Check sheet for the modelled part. Datum: model origin and axes. Units: mm. A direction names the side the tool comes from. Give positions to 0.01 mm unless a question says otherwise; leave off trailing zeros. Order: outer loops, then holes, each group sorted by start corner. A loop starts at its lowest first (then second) coordinate and runs counter-clockwise, first axis right, second up.
```python
from build123d import *

# Parameters (mm, degrees)
SZKIC1_W                     = 60
SZKIC1_H                     = 60
DODANIE_WYCI_GNI_CIE1_DEPTH  = 36.75
SFAZOWANIE1_SIZE             = 5
SFAZOWANIE2_SIZE             = 1
OTW_R_POD_RUB_M51_AT_2_COUNT = 2
OTW_R_POD_RUB_M51_AT_2_PITCH = 47.14
OTW_R_POD_RUB_M51_AT_3_COUNT = 2
OTW_R_POD_RUB_M51_AT_3_PITCH = 66.66602733
OTW_R_POD_RUB_M51_AT_4_COUNT = 2
OTW_R_POD_RUB_M51_AT_4_PITCH = 47.14


with BuildPart() as part:
    # Szkic1 → Dodanie-wyciągnięcie1 (new, symmetric)
    with BuildSketch(Plane(origin=(0, 0, 0), x_dir=(1, 0, 0), z_dir=(0, 1, 0))):
        Rectangle(SZKIC1_W, SZKIC1_H)
    extrude(amount=DODANIE_WYCI_GNI_CIE1_DEPTH, both=True)

    # Szkic2 → Wycięcie-obrót1 (revolve, cut)
    with BuildSketch(Plane.XY, mode=Mode.PRIVATE) as wyci_cie_obr_t1_sk:
        Polygon((29, 4.017949192), (30, 5.75), (36.080330081, 16.281440627), (59, 16.281440627), (59, -27.714101615), (30, -27.714101615), (29, -25.982050808), align=None)
    revolve(wyci_cie_obr_t1_sk.sketch.rotate(Axis((0, 0, 0), (0, 1, 0)), 90), axis=Axis((0, 0, 0), (0, 1, 0)), mode=Mode.SUBTRACT)

    # Sfazowanie1
    sfazowanie1_edges = [part.edges().sort_by_distance(p)[0] for p in [
        (30, -32.232050808, 30),
        (-30, -32.232050808, 30),
        (-30, -32.232050808, -30),
        (30, -32.232050808, -30),
        (30, 26.515720314, 30),
        (-30, 26.515720314, 30),
        (-30, 26.515720314, -30),
        (30, 26.515720314, -30),
    ]]
    chamfer(sfazowanie1_edges, length=SFAZOWANIE1_SIZE)

    # Szkic4 → Wycięcie-obrót3 (revolve, cut)
    with BuildSketch(Plane.XY, mode=Mode.PRIVATE) as wyci_cie_obr_t3_sk:
        Polygon((0, 36.75), (19.05, 36.75), (19.05, 31.75), (4, 31.75), (4, 16.75), (0, 16.75), align=None)
    revolve(wyci_cie_obr_t3_sk.sketch.rotate(Axis((0, 0, 0), (0, 1, 0)), 90), axis=Axis((0, 0, 0), (0, 1, 0)), mode=Mode.SUBTRACT)

    # Szkic5 → Obrót1 (revolve)
    with BuildSketch(Plane(origin=(0, 0, 0), x_dir=(0, 0, -1), z_dir=(1, 0, 0)), mode=Mode.PRIVATE) as obr_t1_sk:
        Polygon((0, -36.75), (20, -36.75), (20, -39.25), (9, -39.25), (9, -40.75), (7, -40.75), (7, -71.75), (0, -71.75), align=None)
    revolve(obr_t1_sk.sketch.rotate(Axis((0, 0, 0), (0, -1, 0)), 180), axis=Axis((0, 0, 0), (0, -1, 0)))

    # Sfazowanie2
    sfazowanie2_edges = [part.edges().sort_by_distance(p)[0] for p in [
        (0, -71.75, -7),
    ]]
    chamfer(sfazowanie2_edges, length=SFAZOWANIE2_SIZE)

    # Szkic7 → Otwór pod śrubę M51 (revolve, cut)
    with BuildSketch(Plane(origin=(23.57, -36.75, -23.57), x_dir=(0, 0, -1), z_dir=(1, 0, 0))):
        Polygon((0, 0), (0, 12.652366702), (2.75, 11), (2.75, 0), align=None)
    otw_r_pod_rub_m51 = revolve(axis=Axis((23.57, -43.1, -23.57), (0, 1, 0)), mode=Mode.SUBTRACT)

    # Otwór pod śrubę M51 at 2: Otwór pod śrubę M51 ×2
    with Locations(*[(-i * OTW_R_POD_RUB_M51_AT_2_PITCH, 0, 0) for i in range(1, OTW_R_POD_RUB_M51_AT_2_COUNT)]):
        add(otw_r_pod_rub_m51, mode=Mode.SUBTRACT)

    # Otwór pod śrubę M51 at 3: Otwór pod śrubę M51 ×2
    with Locations(*[Vector(-0.7071067811865477, 0, 0.7071067811865475) * (i * OTW_R_POD_RUB_M51_AT_3_PITCH) for i in range(1, OTW_R_POD_RUB_M51_AT_3_COUNT)]):
        add(otw_r_pod_rub_m51, mode=Mode.SUBTRACT)

    # Otwór pod śrubę M51 at 4: Otwór pod śrubę M51 ×2
    with Locations(*[(0, 0, i * OTW_R_POD_RUB_M51_AT_4_PITCH) for i in range(1, OTW_R_POD_RUB_M51_AT_4_COUNT)]):
        add(otw_r_pod_rub_m51, mode=Mode.SUBTRACT)

    # Lustro1: Otwór pod śrubę M51 across plane
    add(otw_r_pod_rub_m51.mirror(Plane.ZX), mode=Mode.SUBTRACT)

    # Lustro1 copy 1 sketch → Lustro1 copy 1 (revolve, cut)
    with BuildSketch(Plane(origin=(-23.57, 36.75, -23.57), x_dir=(0, 0, -1), z_dir=(1, 0, 0))):
        Polygon((0, 0), (0, -12.652366702), (2.75, -11), (2.75, 0), align=None)
    revolve(axis=Axis((-23.57, 43.1, -23.57), (0, 1, 0)), mode=Mode.SUBTRACT)

    # Lustro1 copy 2 sketch → Lustro1 copy 2 (revolve, cut)
    with BuildSketch(Plane(origin=(-23.57, 36.75, 23.57), x_dir=(0, 0, -1), z_dir=(1, 0, 0))):
        Polygon((0, 0), (0, -12.652366702), (2.75, -11), (2.75, 0), align=None)
    revolve(axis=Axis((-23.57, 43.1, 23.57), (0, 1, 0)), mode=Mode.SUBTRACT)

    # Lustro1 copy 3 sketch → Lustro1 copy 3 (revolve, cut)
    with BuildSketch(Plane(origin=(23.57, 36.75, 23.57), x_dir=(0, 0, -1), z_dir=(1, 0, 0))):
        Polygon((0, 0), (0, -12.652366702), (2.75, -11), (2.75, 0), align=None)
    revolve(axis=Axis((23.57, 43.1, 23.57), (0, 1, 0)), mode=Mode.SUBTRACT)


solid = part.part
```
(1) Material ranges on L1, parallel to X at y = 33, z = -23.57; L2, parallel to X at y = -30, z = 24, recorded low to high.
Response values:
L1: x = -30 to -26.32, -20.82 to 20.82, 26.32 to 30
L2: x = -30 to -26.29, -20.85 to 20.85, 26.29 to 30
(2) Cross-section at A-A on y = -8.5. Enter the section's corners in (x, z), then the cut area to 3 significant figures.
Response values:
outline: circle Ø58 at (0, 0)
area: 2,640 mm2
(3) Set-up check for faces 1 (the face through (20.843, -32.295, -23.212)), 2 (the face through (0, -71.75, 0)), 3 (the face through (-27, 16.281, -27)), 4 (the face through (-14, 36.75, -14)), 5 (the face through (-5, 31.75, 0)): record each of +Z, -Z, +X, -X, +Y, -Y from which the full face is reachable in a straight line by a thin tool's end or side.
Response values:
face 1: -Y
face 2: +Z, -Z, +X, -X, -Y
face 3: -Z, -X
face 4: +Z, -Z, +X, -X, +Y
face 5: +Y
(4) Gauge pin test, flat ends, axial feed: pin 1 Ø12 at (x, z) = (17.5, -12) entering from -Y; pin 2 Ø5 at (x, z) = (27.5, 26.5) entering from -Y; pin 3 Ø3.5 at (x, z) = (-23.57, -23.57) entering from +Y; pin 4 Ø20 at (x, z) = (10, -3) entering from -Y. Record the tip position at first contact, or that the pin passes through.
Response values:
pin 1: stops at y = -39.25
pin 2: stops at y = -36.75
pin 3: stops at y = 25.15
pin 4: stops at y = -71.75
(5) Release check for a two-part mould opening along X. For faces 6 (the face through (18.597, 34.215, 4.13)), 7 (the face through (-27, 26, 28)), 8 (the face through (0, -32, 30)) record: released by +X, released by -X, zero draft, split by the parting line, or undercut.
Response values:
face 6: undercut
face 7: released by -X
face 8: zero draft
